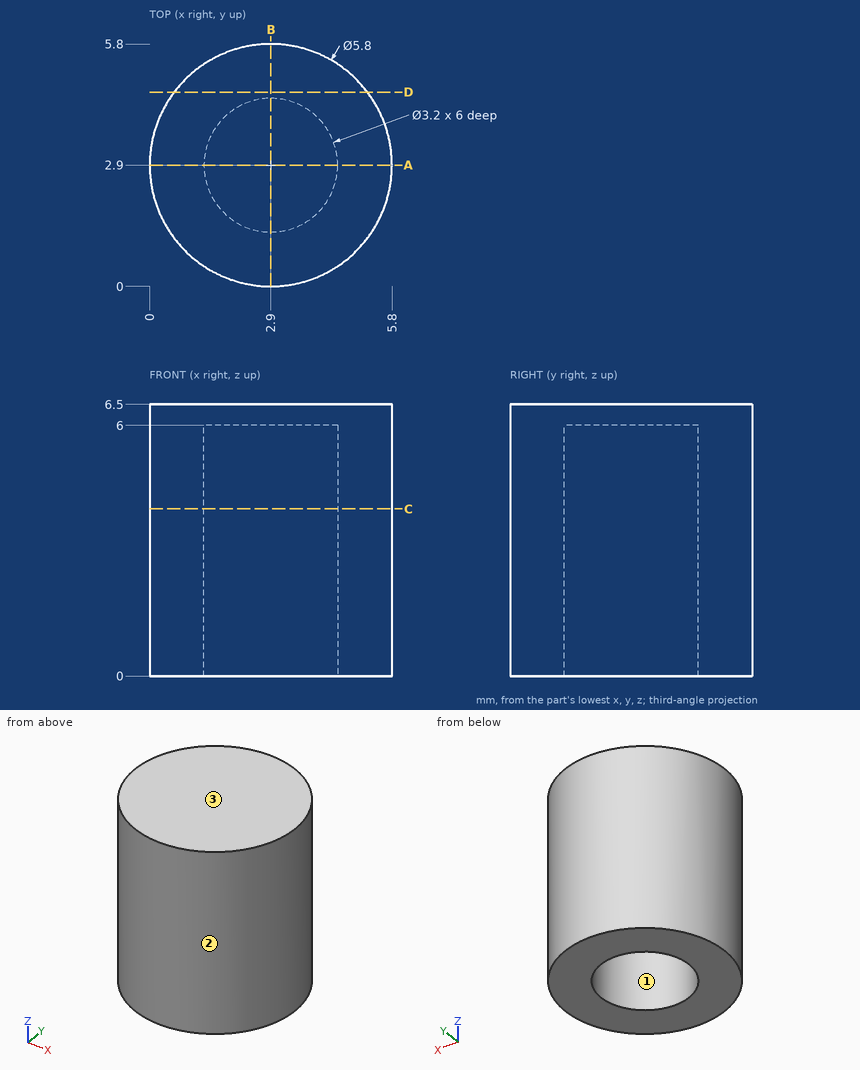
The drawing under review shows one solid part. Ordinate dimensions are in mm from its lowest x, y, z. Round coordinates to 2 decimals unless told otherwise and drop trailing zeros. Loops run counter-clockwise (first coordinate to the right, second up) from the corner with the lowest first, then second, coordinate; pieces in that order, holes last. Notation, with made-up numbers: M 77.5,-25.75 L 94.5,-25.75 A15 cw 94.5,-13.75 Z; hole C 84,54.25 d3. An arc over 180 degrees is marked long. Answer as CSV lines item,"result". Start each with the question number.
Item 1: Consider section A-A (y = 2.9). Write out the cut boundary in (x, z), then the cut area to 3 significant figures.
Item 2: Insertion check: P1, Ø1.6, axis at x = 3, y = 3.5, coming from the -Z side; P2, Ø1, axis at x = 4.5, z = 0.5, coming from the +Y side; P3, Ø3, axis at x = 4.5, z = 1, coming from the -Y side. Each pin has a flat end and moves straight along its axis. Give the tip position at first contact, or say it passes through.
Item 3: Consider section D-D (y = 4.65). Write out the cut boundary in (x, z), then the cut area to 3 significant figures.
Item 4: Wall thickness on line 1 (Y direction, x = 2.9, z = 3.25); line 2 (Z direction, x = 4.1, y = 3.65); line 3 (Y direction, x = 1.65, z = 4): over which ranges is each line inside the solid? List them lowest first. Write a range as [from, to].
Item 5: Consider section C-C (z = 4). Write out the cut boundary in (x, y), then the cut area to 3 significant figures.
Item 6: Mouldability with a two-part tool opening along X and no side actions: class the marked faces 1, 2 and 3 as released by +X, released by -X, zero draft, split by the parting line, or undercut.
Answer:
1,outline,"M 0,0 L 1.3,0 L 1.3,6 L 4.5,6 L 4.5,0 L 5.8,0 L 5.8,6.5 L 0,6.5 Z"
1,area,"18.5 mm^2"
2,P1,"stops at z = 6"
2,P2,"stops at y = 5.58"
2,P3,"stops at y = 0"
3,outline,"M 0.59,0 L 5.21,0 L 5.21,6.5 L 0.59,6.5 Z"
3,area,"30.1 mm^2"
4,line 1,"y = [0, 1.3], [4.5, 5.8]"
4,line 2,"z = [6, 6.5]"
4,line 3,"y = [0.28, 1.9], [3.9, 5.52]"
5,outline,"C 2.9,2.9 d5.8; hole C 2.9,2.9 d3.2"
5,area,"18.4 mm^2"
6,face 1,"undercut"
6,face 2,"split by the parting line"
6,face 3,"zero draft"
